Autodesk Inventor part; units mm, degrees
ref_plane "ip_st_1_XY" through (0, 0, 0) normal (1, 0, 0) x (0, 0, -1)
ref_plane "ip_st_1_YZ" through (0, 0, 0) normal (0, 0, -1) x (0, 1, 0)
ref_plane "ip_st_1_ZX" through (0, 0, 0) normal (0, 1, 0) x (1, 0, 0)
sketch "Sketch_1" plane through (0, 0, 0) normal (0, 0, 1) x (1, 0, 0)
  line L0 (4, 0) -> (0, 0)
  line L1 (0, 5.45) -> (0.25, 5.45)
  line L2 (0.25, 5.45) -> (0.25, 5.095)
  line L3 (0.25, 5.095) -> (1.3247, 5.095)
  arc A0 (2.6753, 5.095) -> (1.3247, 5.095) centre (2, 4.5) ccw
  line L4 (2.6753, 5.095) -> (3.75, 5.095)
  line L5 (3.75, 5.095) -> (3.75, 5.45)
  line L6 (3.75, 5.45) -> (4, 5.45)
  line L7 (4, 5.45) -> (4, 6.65)
  arc A1 (4, 6.65) -> (3.85, 6.8) centre (3.85, 6.65) ccw
  line L8 (3.85, 6.8) -> (3.2, 6.8)
  line L9 (3.2, 6.8) -> (3.2, 6)
  line L10 (3.2, 6) -> (0.15, 6)
  arc A2 (0.15, 6) -> (0, 5.85) centre (0.15, 5.85) ccw
  line L11 (0, 5.85) -> (0, 5.45)
revolve "Revolution1" add sketch "Sketch_1" angle 360 about axis through (4, 0, 0) along (1, 0, 0)
ref_plane "ip_st_1_XY" through (0, 0, 0) normal (1, 0, 0) x (0, 0, -1)
ref_plane "ip_st_1_YZ" through (0, 0, 0) normal (0, 0, -1) x (0, 1, 0)
ref_plane "ip_st_1_ZX" through (0, 0, 0) normal (0, 1, 0) x (1, 0, 0)
ref_plane "ip_st_2_XY" through (3.75, 0, 0) normal (-1, 0, 0) x (0, 0, -1)
ref_plane "ip_st_2_YZ" through (3.75, 0, 0) normal (0, 0, -1) x (0, -1, 0)
ref_plane "ip_st_2_ZX" through (3.75, 0, 0) normal (0, -1, 0) x (-1, 0, 0)
properties part number "MF126ZZ Outer Ring"
Input: part model. Units: mm. Frame: model coordinates. A direction names the side the tool comes from. Coordinates: 2 decimals unless noted, no trailing zeros. Loops run counter-clockwise (first coordinate to the right, second up) from the corner with the lowest first, then second, coordinate; pieces in that order, holes last.
(1) Section D-D on x = 2.45. Return the cut outline in (y, z), then the cut area to 3 significant figures.
(2) Pull-direction query (Y, two-part tool) for faces 1 (the face through (3.22, -1.104, -4.974)), 2 (the face through (3.2, 4, -5)), 3 (the face through (0.795, -1.104, -4.974)), 4 (the face through (3.52, -1.47, 6.64)); classes: released by +Y, released by -Y, zero draft, split by the parting line, or undercut.
(3) First-contact query: pin 1 Ø1.5 at (y, z) = (1, -4.5) entering from -X. Flat tip, straight axial feed; report the tip coordinate or a pass-through.
(4) Section A-A on z = 0. Return the cut outline in (x, y) (3 decimals).
(5) Set-up query: faces 5 (the face through (0, 4, -4)), 6 (the face through (2, -6, 0)). Return all of +Z, -Z, +X, -X, +Y, -Y with unobstructed straight access to the full face (end or side cutting, diameter ignored); none if empty.
(6) Material intervals for probe 1 along Z at (x, y) = (3.8, 0); probe 2 along Z at (x, y) = (3, 0) (3 decimals); probe 3 along X at (y, z) = (3.5, 5.5), sorted ascending.
(7) Section C-C on x = 0.6. Return the cut outline in (y, z) (3 decimals).
Data:
1. outline: circle Ø12 at (0, 0); hole circle Ø10.56 at (0, 0)
1. area: 25.5 mm2
2. face 1: undercut
2. face 2: zero draft
2. face 3: undercut
2. face 4: split by the parting line
3. pin 1: stops at x = 0.25
4. outline: (0, -5.85) arc R0.15 ccw to (0.15, -6) - (3.2, -6) - (3.2, -6.8) - (3.85, -6.8) arc R0.15 ccw to (4, -6.65) - (4, -5.45) - (3.75, -5.45) - (3.75, -5.095) - (2.675, -5.095) arc R0.9 cw to (1.325, -5.095) - (0.25, -5.095) - (0.25, -5.45) - (0, -5.45) - close; (0, 5.45) - (0.25, 5.45) - (0.25, 5.095) - (1.325, 5.095) arc R0.9 cw to (2.675, 5.095) - (3.75, 5.095) - (3.75, 5.45) - (4, 5.45) - (4, 6.65) arc R0.15 ccw to (3.85, 6.8) - (3.2, 6.8) - (3.2, 6) - (0.15, 6) arc R0.15 ccw to (0, 5.85) - close
5. face 5: +Z, -Z, -X, +Y, -Y
5. face 6: -X
6. probe 1: z = -6.8 to -5.45, 5.45 to 6.8
6. probe 2: z = -6 to -5.095, 5.095 to 6
6. probe 3: x = 3.2 to 4
7. outline: circle Ø12 at (0, 0); hole circle Ø10.19 at (0, 0)
